Design review of the part shown in the three views and the two pictorial views. Dimensions are in mm from the part's minimum x, y and z. Round coordinates to 2 decimals unless told otherwise and drop trailing zeros. Write each loop counter-clockwise with the first axis right and the second up, starting at its lowest first coordinate (ties: lowest second). Pieces come first, ordered by that corner, then holes. Notation, with made-up numbers: (-18.5, 46) -> (26.5, 46) arc R19 ccw to (26.5, 71) -> close; hole circle Ø7 at (47.25, 86). An arc over 180 degrees is marked (long way). Answer as a JSON object with one key per item and string values. Group by question number.
1) We need section A-A, the plane y = 1.05. Write out the cut boundary in (x, z).
2) We need section C-C, the plane x = 34.5. Write out the cut boundary in (y, z), then the cut area to 3 significant figures.
3) To check wall thickness, follow probe 1 along Z at (x, y) = (20, 1.5); probe 2 along Z at (x, y) = (46.5, 1.9); probe 3 along X at (y, z) = (4.4, 18). State the ranges of each line that lie inside material, in increasing order. Write a range as [from, to].
4) Insertion check: pin 1 Ø2 at (x, y) = (25, 3) entering from +Z. The pin has a flat end and moves straight along its axis. Give the tip position at first contact, or say it passes through.
5) We need section B-B, the plane z = 41.5. Write out the cut boundary in (x, y), then the cut area to 3 significant figures.
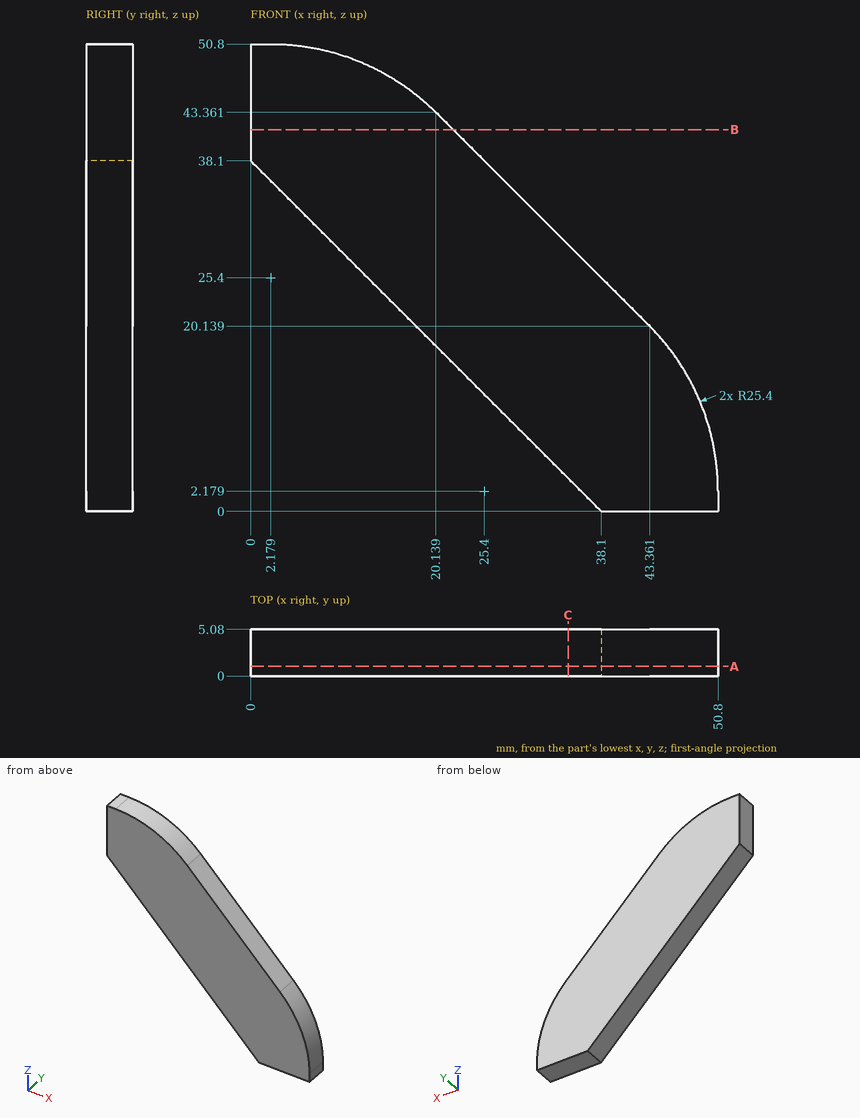
Here are the results:
{
 "1": {"outline": "(0, 38.1) -> (38.1, 0) -> (50.8, 0) -> (50.8, 2.18) arc R25.4 ccw to (43.36, 20.14) -> (20.14, 43.36) arc R25.4 ccw to (2.18, 50.8) -> (0, 50.8) -> close"},
 "2": {"outline": "(0, 3.6) -> (5.08, 3.6) -> (5.08, 29) -> (0, 29) -> close", "area": "129 mm^2"},
 "3": {"probe 1": "z = [18.1, 43.5]", "probe 2": "z = [0, 16.32]", "probe 3": "x = [20.1, 45.27]"},
 "4": {"pin 1": "stops at z = 39.5"},
 "5": {"outline": "(0, 0) -> (22, 0) -> (22, 5.08) -> (0, 5.08) -> close", "area": "112 mm^2"}
}
